Autodesk Inventor part; units mm, degrees
ref_plane "YZ Plane" through (0, 0, 0) normal (1, 0, 0) x (0, 1, 0)
ref_plane "XZ Plane" through (0, 0, 0) normal (0, 1, 0) x (-1, 0, 0)
ref_plane "XY Plane" through (0, 0, 0) normal (0, 0, 1) x (1, 0, 0)
sketch "Sketch1" plane through (0, 0, 0) normal (0, 0, 1) x (1, 0, 0)
  line L0 (0, 0) -> (76.2, 0)
  line L1 (76.2, 0) -> (76.2, 203.2)
  line L2 (76.2, 203.2) -> (0, 203.2)
  line L3 (0, 203.2) -> (0, 0)
  line L4 (0, 203.2) -> (-406.4, 203.2) construction
  line L5 (0, 203.2) -> (-1016, 256.4463)
  line L6 (0, 0) -> (-1016, 0)
  line L7 (-1016, 0) -> (-1016, 256.4463)
  dimension "d0" = 203.2
  dimension "d1" = 76.2
  dimension "d2" = 3
  dimension "d3" = 1016
extrude "Extrusion1" add sketch "Sketch1" along normal blind 11.938
properties part number "Outlet Support Leg Proto 1" material "Wood (Oak)"
CAD build for the part. Positions are in the model's coordinates, mm. Coordinates: 2 decimals unless noted, no trailing zeros. Write each loop counter-clockwise with the first axis right and the second up, starting at its lowest first coordinate (ties: lowest second). Pieces come first, ordered by that corner, then holes. Notation, with made-up numbers: M 45.25,23.25 L 92.25,23.25 A22 ccw 92.25,43.25 Z; hole C 21.5,87 d1. An arc over 180 degrees is marked long. Return JSON: item names as keys, results as strings.
Item 1: Slice it at B-B, the plane y = 228. Write the cut outline in (x, z), and give its area (3 significant figures).
Findings below:
{"outline": "M -1016,0 L -473.21,0 L -473.21,11.94 L -1016,11.94 Z", "area": "6,480 mm2"}
Item 2: Slice it at A-A, the plane z = 4.5. Write the cut outline in (x, y), and give its area (3 significant figures).
Findings below:
{"outline": "M -1016,0 L 76.2,0 L 76.2,203.2 L 0,203.2 L -1016,256.45 Z", "area": "249,000 mm2"}
Item 3: Drop a flat-ended pin along its axis: pin 1 Ø2 at (x, z) = (-665.5, 5) entering from +Y. Give the stop position or say it passes through.
Findings below:
{"pin 1": "stops at y = 238.13"}
Item 4: Slice it at C-C, the plane x = -67. Write the cut outline in (y, z).
Findings below:
{"outline": "M 0,0 L 206.71,0 L 206.71,11.94 L 0,11.94 Z"}
Item 5: Probe line 1 (Y direction, x = 23.5, z = 2.5); line 2 (Y direction, x = -259, z = 9.25). List the from-to ranges inside material, lowest first. Write a range as from..to.
Findings below:
{"line 1": "y = 0..203.2", "line 2": "y = 0..216.77"}
